Geometry: final body of the model. Coordinates: model frame, mm. Face numbers are marked on the shaded views. Round coordinates to 2 decimals unless told otherwise and drop trailing zeros. Loops run counter-clockwise (first coordinate to the right, second up) from the corner with the lowest first, then second, coordinate; pieces in that order, holes last. Notation, with made-up numbers: (14.5, 88.5) - (37.5, 88.5) arc R23 cw to (37.5, 105.5) - close; hole circle Ø7 at (38, 38.25). An arc over 180 degrees is marked (long way). Write item = value, one per line. Start each with the question number.
Item 1: Section A-A (x = 0). Return loops of the section in (y, z).
Item 2: Section D-D (z = 35). Return loops of the section in (x, y).
Item 3: Line query: line 1 (Y direction, x = 0, z = 54); line 2 (Y direction, x = 0, z = 16); line 3 (Z direction, x = 0, y = 10.3). Output: solid intervals per line, ascending. Write a range as from..to.
Item 4: Section B-B (y = 0). Return loops of the section in (x, z).
Item 5: First-contact query: pin 1 (12 mm diameter, centred on x = 7.5, y = 9.5, fed in from -Z); pin 2 (8 mm diameter, centred on x = -4.5, z = 16.5, fed in from -Y); pin 3 (10 mm diameter, centred on y = -7, z = 10, fed in from +X); pin 4 (1 mm diameter, centred on x = 4, z = 33.5, fed in from +Y). Flat tips, straight axial feed; report the tip coordinate or a pass-through.
Item 6: Section C-C (z = 46). Return loops of the section in (x, y), plus the area to 3 significant figures.
Item 7: Draft query along Y for the marked faces 1, 2 and 3. Return one class per face: pulls with the +Y half, pulls with the -Y half, needs draft (parallel to the pull), parting line crosses it, or undercut.
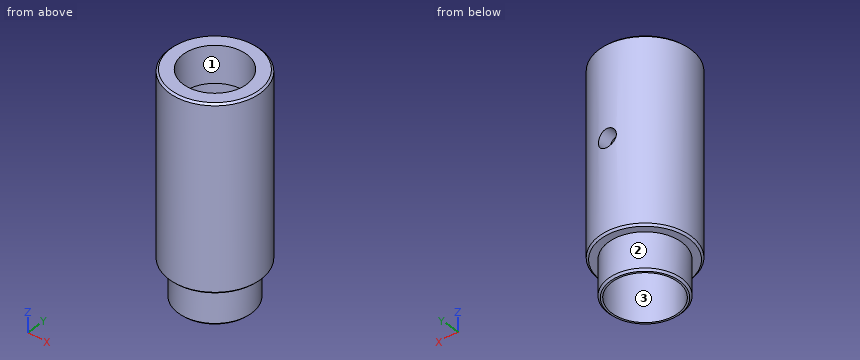
Autodesk Inventor part; units mm, degrees
ref_plane "Arbeitsebene1" through (0, 12.5, 0) normal (0, 1, 0) x (-1, 0, 0)
ref_plane "YZ Plane" through (0, 0, 0) normal (1, 0, 0) x (0, 1, 0)
ref_plane "XY Plane" through (0, 0, 0) normal (0, 0, 1) x (1, 0, 0)
sketch "Skizze1" plane through (0, 0, 0) normal (0, 0, 1) x (1, 0, 0)
  line L0 (-14, 0) -> (14, 0)
  line L1 (0, -14) -> (0, 14)
  circle A0 centre (0, 0) radius 10
  dimension "d0" = 20
extrude "Extrusion1" add sketch "Skizze1" along normal blind 10
sketch "Skizze2" plane through (0, 0, 10) normal (0, 0, 1) x (1, 0, 0)
  circle A0 centre (0, 0) radius 12.5
  dimension "d3" = 25
extrude "Extrusion2" add sketch "Skizze2" along normal blind 50
sketch "Skizze3" plane through (0, 0, 60) normal (0, 0, 1) x (1, 0, 0)
  circle A0 centre (0, 0) radius 10
  dimension "d6" = 20
extrude "Extrusion3" add sketch "Skizze3" along normal blind 10
thread "Gewinde1"
thread "Gewinde2"
sketch "Skizze4" plane through (0, 0, 0) normal (0, 0, -1) x (-1, 0, 0)
  circle A0 centre (0, 0) radius 9
  dimension "d13" = 18
extrude "Extrusion4" cut sketch "Skizze4" against normal blind 70
ref_plane "Arbeitsebene1" through (0, 12.5, 0) normal (0, 1, 0) x (-1, 0, 0)
sketch "Skizze5" plane through (0, 0, 0) normal (0, 1, 0) x (-1, 0, 0)
  point P0 (0, 0)
sketch "Skizze6" plane through (0, 12.5, 0) normal (0, 1, 0) x (-1, 0, 0)
  circle A0 centre (0, 35) radius 2.5
  point P0 (0, 0)
  dimension "d17" = 35
  dimension "d18" = 5
extrude "Extrusion5" cut sketch "Skizze6" against normal blind 5
chamfer "Fase1" distance 0.5 angle 45 4 edges at (-10, 0, 0) (-10, 0, 70) (-12.5, 0, 10) (-12.5, 0, 60)
sketch "Skizze7" plane through (0, 0, 0) normal (0, 0, -1) x (-1, 0, 0)
  point P0 (0, 0)
  point P1 (0, 0)
sketch "Skizze8" plane through (0, 0, 70) normal (0, 0, 1) x (1, 0, 0)
  circle A0 centre (0, 0) radius 9
  circle A1 centre (0, 0) radius 11.265
extrude "Extrusion6" cut sketch "Skizze8" against normal blind 10 contours A0 | A1
sketch "Skizze9" plane through (0, 0, 60) normal (0, 0, 1) x (1, 0, 0)
  circle A0 centre (0, 0) radius 9
extrude "Extrusion7" add sketch "Skizze9" against normal blind 10
sketch "Skizze10" plane through (0, 0, 60) normal (0, 0, 1) x (1, 0, 0)
  point P0 (0, 0)
hole "Bohrung1" at (0, 0, 60) direction (0, 0, -1) diameter 17.294 end through all
properties part number "VentilNukleator"
Taken from the geometry:
q1.outline = (-12.5, 10.5) - (-12, 10) - (-10, 10) - (-10, 0.5) - (-9.5, 0) - (-9, 0) - (-9, 50) - (-8.65, 50) - (-8.65, 60) - (-12, 60) - (-12.5, 59.5) - close; (8.65, 50) - (9, 50) - (9, 37.5) - (12.5, 37.5) - (12.5, 59.5) - (12, 60) - (8.65, 60) - close; (9, 0) - (9.5, 0) - (10, 0.5) - (10, 10) - (12, 10) - (12.5, 10.5) - (12.5, 32.5) - (9, 32.5) - close
q2.outline = (-2.5, 8.65) - (-2.5, 12.25) arc R12.5 ccw (long way) to (2.5, 12.25) - (2.5, 8.65) arc R9 cw (long way) to start
q3.line_1 = -12.5..-8.65, 8.65..12.5
q3.line_2 = -12.5..-9, 9..12.5
q3.line_3 = 10..32.5, 37.5..60
q4.outline = (-12.5, 10.5) - (-12, 10) - (-10, 10) - (-10, 0.5) - (-9.5, 0) - (-9, 0) - (-9, 50) - (-8.65, 50) - (-8.65, 60) - (-12, 60) - (-12.5, 59.5) - close; (8.65, 50) - (9, 50) - (9, 0) - (9.5, 0) - (10, 0.5) - (10, 10) - (12, 10) - (12.5, 10.5) - (12.5, 59.5) - (12, 60) - (8.65, 60) - close
q5.pin_1 = 0
q5.pin_2 = -12.49
q5.pin_3 = 12.33
q5.pin_4 = 12
q6.outline = circle Ø25 at (0, 0); hole circle Ø18 at (0, 0)
q6.area = 236 mm^2
q7.face_1 = undercut
q7.face_2 = parting line crosses it
q7.face_3 = undercut
